CAD build for the part. Positions are in the model's coordinates, mm. Give positions to 0.01 mm unless a question says otherwise; leave off trailing zeros. Write each loop counter-clockwise with the first axis right and the second up, starting at its lowest first coordinate (ties: lowest second). Pieces come first, ordered by that corner, then holes. Notation, with made-up numbers: (2, 10.5) - (45, 10.5) arc R36 ccw to (45, 45.5) - close; hole circle Ø7 at (-8.5, 4.25). An arc over 180 degrees is marked (long way). Answer as a JSON object with one key per item and string values.
from build123d import *

# Parameters (mm, degrees)
EXTRUDE1_DEPTH  = 1.524
SKETCH2_R       = 2.413
EXTRUDE2_DEPTH  = 2.524
LPATTERN1_COUNT = 3
LPATTERN1_PITCH = 12.7


with BuildPart() as part:
    # Sketch1 → Extrude1 (new body)
    with BuildSketch(Plane.XY):
        with BuildLine():
            Line((-12.7, -6.35), (12.7, -6.35))
            ThreePointArc((12.7, -6.35), (19.05, 0), (12.7, 6.35))
            Line((12.7, 6.35), (-12.7, 6.35))
            ThreePointArc((-12.7, 6.35), (-19.05, 0), (-12.7, -6.35))
        make_face()
    extrude(amount=EXTRUDE1_DEPTH)

    # Sketch2 → Extrude2 (cut, through all)
    with BuildSketch(Plane.XY.offset(1.524)):
        with Locations((-12.7, 0)):
            Circle(SKETCH2_R)
    extrude2 = extrude(amount=-EXTRUDE2_DEPTH, mode=Mode.SUBTRACT)

    # LPattern1: Extrude2 ×3
    with Locations(*[(i * LPATTERN1_PITCH, 0, 0) for i in range(1, LPATTERN1_COUNT)]):
        add(extrude2, mode=Mode.SUBTRACT)


solid = part.part
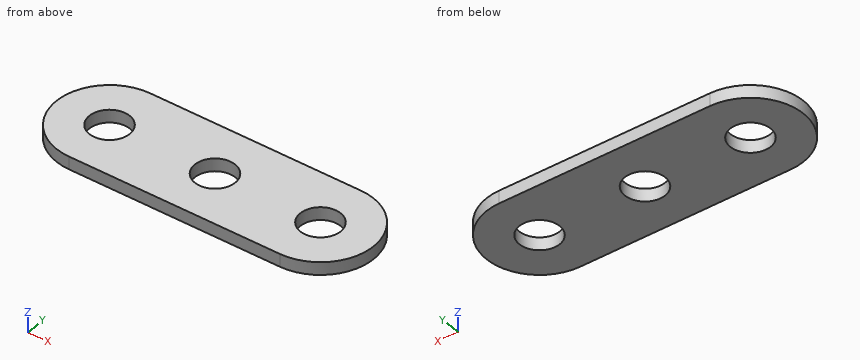
Item 1: Cut at D-D (x = -14). Give the cut face in (y, z), and give its area (3 significant figures).
Entries:
{"outline": "(-6.22, 0) - (-2.03, 0) - (-2.03, 1.52) - (-6.22, 1.52) - close; (2.03, 0) - (6.22, 0) - (6.22, 1.52) - (2.03, 1.52) - close", "area": "12.7 mm2"}
Item 2: Cut at A-A (y = 0). Give the cut face in (x, z).
Entries:
{"outline": "(-19.05, 0) - (-15.11, 0) - (-15.11, 1.52) - (-19.05, 1.52) - close; (-10.29, 0) - (-2.41, 0) - (-2.41, 1.52) - (-10.29, 1.52) - close; (2.41, 0) - (10.29, 0) - (10.29, 1.52) - (2.41, 1.52) - close; (15.11, 0) - (19.05, 0) - (19.05, 1.52) - (15.11, 1.52) - close"}
Item 3: Cut at C-C (z = 0.95). Give the cut face in (x, y).
Entries:
{"outline": "(-12.7, -6.35) - (12.7, -6.35) arc R6.35 ccw to (12.7, 6.35) - (-12.7, 6.35) arc R6.35 ccw to start; hole circle Ø4.83 at (-12.7, 0); hole circle Ø4.83 at (0, 0); hole circle Ø4.83 at (12.7, 0)"}
Item 4: Cut at B-B (x = 0). Give the cut face in (y, z).
Entries:
{"outline": "(-6.35, 0) - (-2.41, 0) - (-2.41, 1.52) - (-6.35, 1.52) - close; (2.41, 0) - (6.35, 0) - (6.35, 1.52) - (2.41, 1.52) - close"}
Item 5: Probe line 1 (X direction, y = 1.75, z = 0.95); line 2 (Y direction, x = -12.7, z = 0.4); line 3 (X direction, y = 0.5, z = 1.2). List the from-to ranges inside material, lowest first. Write a range as from..to.
Entries:
{"line 1": "-18.8..-14.36, -11.04..-1.66, 1.66..11.04, 14.36..18.8", "line 2": "-6.35..-2.41, 2.41..6.35", "line 3": "-19.03..-15.06, -10.34..-2.36, 2.36..10.34, 15.06..19.03"}
